Read the model definition and answer for the solid it produces. Units are mm, in the model's axes. Coordinates: 2 decimals unless noted, no trailing zeros. Loops run counter-clockwise (first coordinate to the right, second up) from the corner with the lowest first, then second, coordinate; pieces in that order, holes last.
Q1. The mould has two halves that part along X. Classify faces 1 (the face through (-37.958, -181.576, 12.211)), 2 (the face through (-20.576, -233.407, 13.189)), 3 (the face through (149.356, 29.252, 12.211)): pulls with the +X half, pulls with the -X half, needs draft (parallel to the pull), parting line crosses it, or undercut.
Q2. Section D-D (x = 630) is taken. Give the vertices of the cut face in (y, z) (3 decimals), then the cut area to 3 significant figures.
Q3. Straight lines are drawn through the part: line 1 (Y direction, x = -30, z = -12.5) (3 decimals); line 2 (Y direction, x = 114, z = 28); line 3 (Y direction, x = 256, z = -18.5). For each, find the intervals that lie inside material, in ascending order.
Q4. Section A-A (x = 137) is taken. Give the vertices of the cut face in (y, z) (3 decimals), then the cut area to 3 significant figures.
Q5. Section B-B (z = -8) is taken. Give the vertices of the cut face in (x, y).
Q6. Flat-ended cylindrical pins translate along their axes: P1, Ø1.5, axis at y = -31.5, z = -11, coming from the -X side; P2, Ø4, axis at x = 796.5, z = 16, coming from the -Y side; P3, Ø1, axis at y = -40, z = 5, coming from the -X side. Find the tip coordinate at first contact, or state that the pin passes through.
Q7. Section C-C (y = -75) is taken. Give the vertices of the cut face in (x, z) (3 decimals), then the cut area to 3 significant figures.
Autodesk Inventor part; units mm, degrees
ref_plane "YZ Plane" through (0, 0, 0) normal (1, 0, 0) x (0, 1, 0)
ref_plane "XZ Plane" through (0, 0, 0) normal (0, 1, 0) x (-1, 0, 0)
ref_plane "XY Plane" through (0, 0, 0) normal (0, 0, 1) x (1, 0, 0)
ref_plane "Work Plane1" through (0, 0, -22.225) normal (0, 0, -1) x (-1, 0, 0)
sketch "Sketch1" plane through (0, 0, -22.225) normal (0, 0, -1) x (-1, 0, 0)
  arc A0 (88.9626, 123.799) -> (43.8693, -146.1511) centre (0.2092, -0.1167) ccw
  line L0 (104.0584, 214.2592) -> (-870.0682, 186.8193)
  line L1 (-870.0682, 186.8193) -> (-996.5964, 89.8924)
  line L2 (-996.5964, 89.8924) -> (27.3448, -245.173)
  line L3 (104.0584, 214.2592) -> (88.9626, 123.799)
  line L4 (27.3448, -245.173) -> (43.8693, -146.1511)
extrude "Extrusion1" add sketch "Sketch1" against normal blind 69.85
fillet "Fillet1" radius 25.4 1 edges at (-104.0584, 214.2592, 12.7)
fillet "Fillet2" radius 25.4 1 edges at (-27.3448, -245.173, 12.7)
fillet "Fillet3" radius 25.4 2 edges at (996.5964, 89.8924, 12.7) (870.0682, 186.8193, 12.7)
properties material "Wood (Walnut)"
Numbers:
1. face 1: pulls with the -X half
1. face 2: parting line crosses it
1. face 3: undercut
2. outline: (-30.069, -22.225) - (193.582, -22.225) - (193.582, 47.625) - (-30.069, 47.625) - close
2. area: 15,600 mm2
3. line 1: y = -222.946 to -149.598, 149.365 to 212.173
3. line 2: y = -198.92 to -101.05, 100.82 to 208.12
3. line 3: y = -152.45 to 204.12
4. outline: (-191.394, -22.225) - (-66.494, -22.225) - (-66.494, 47.625) - (-191.394, 47.625) - close; (66.26, -22.225) - (207.469, -22.225) - (207.469, 47.625) - (66.26, 47.625) - close
4. area: 18,600 mm2
5. outline: (-98.98, 183.82) - (-88.96, 123.8) arc R152.42 cw (long way) to (-43.87, -146.15) - (-32.21, -216.02) arc R25.4 ccw to (0.74, -235.98) - (950.78, 74.9) arc R25.4 ccw to (958.33, 119.21) - (876.59, 181.82) arc R25.4 ccw to (861.86, 187.05) - (-73.21, 213.39) arc R25.4 ccw to start
6. P1: stops at x = 148.79
6. P2: stops at y = 23.76
6. P3: stops at x = 146.77
7. outline: (132.549, -22.225) - (492.694, -22.225) - (492.694, 47.625) - (132.549, 47.625) - close
7. area: 25,200 mm2
